Here's how the part is built. I have some questions about the finished solid (model axes, mm). A direction names the side the tool comes from. Coordinates: 2 decimals unless noted, no trailing zeros. Write each loop counter-clockwise with the first axis right and the second up, starting at its lowest first coordinate (ties: lowest second). Pieces come first, ordered by that corner, then holes. Notation, with made-up numbers: M 20,-38.5 L 36,-38.5 A12 cw 36,-18.5 Z; hole C -34.5,-5 d3. An arc over 180 degrees is marked long. Use a Markdown table: item, result.
```python
from build123d import *

# Parameters (mm, degrees)
BOSS_EXTRUDE1_DEPTH       = 46
SKETCH3_W                 = 25
SKETCH3_H                 = 25
BOSS_EXTRUDE2_DEPTH       = 2
SKETCH4_R                 = 1.25
SKETCH4_R_2               = 5
CUT_EXTRUDE1_DEPTH        = 3
FILLET1_R                 = 10
SKETCH5_R                 = 2
CUT_EXTRUDE2_DEPTH        = 26
LPATTERN1_COUNT           = 4
LPATTERN1_PITCH           = 10
LPATTERN1_COPY_1_SKETCH_R = 2
LPATTERN1_COPY_1_DEPTH    = 26
LPATTERN1_COPY_2_SKETCH_R = 2
LPATTERN1_COPY_2_DEPTH    = 26
LPATTERN1_COPY_3_SKETCH_R = 2
LPATTERN1_COPY_3_DEPTH    = 26


with BuildPart() as part:
    # Sketch2 → Boss-Extrude1 (new body)
    with BuildSketch(Plane.XY):
        with BuildLine():
            Line((-12.5, -3.978039328), (12.5, -3.978039328))
            Line((12.5, -3.978039328), (12.468421549, 6.021910812))
            Line((12.468421549, 6.021910812), (10.968421549, 6.021910812))
            ThreePointArc((10.968421549, 6.021910812), (0, 0), (-10.968421549, 6.021910812))
            Line((-10.968421549, 6.021910812), (-12.468421549, 6.021910812))
            Line((-12.468421549, 6.021910812), (-12.5, -3.978039328))
        make_face()
    extrude(amount=BOSS_EXTRUDE1_DEPTH)

    # Sketch3 → Boss-Extrude2 (add)
    with BuildSketch(Plane(origin=(0, 0, 0), x_dir=(-1, 0, 0), z_dir=(0, 0, -1))):
        with Locations((0, 8.521960672)):
            Rectangle(SKETCH3_W, SKETCH3_H)
    extrude(amount=BOSS_EXTRUDE2_DEPTH)

    # Sketch4 → Cut-Extrude1 (cut, through all)
    with BuildSketch(Plane.XY):
        with Locations((-9.5, 13)):
            Circle(SKETCH4_R)
        with Locations((9.5, 13)):
            Circle(SKETCH4_R)
        with Locations((0, 10)):
            Circle(SKETCH4_R_2)
    extrude(amount=-CUT_EXTRUDE1_DEPTH, mode=Mode.SUBTRACT)

    # Fillet1
    fillet1_edges = [part.edges().sort_by_distance(p)[0] for p in [
        (12.5, 21.021960672, -1),
        (-12.5, 21.021960672, -1),
    ]]
    fillet(fillet1_edges, radius=FILLET1_R)

    # Sketch5 → Cut-Extrude2 (cut, through all)
    with BuildSketch(Plane.XZ.offset(3.978039328)):
        with Locations((-8.5, 8)):
            Circle(SKETCH5_R)
    cut_extrude2 = extrude(amount=-CUT_EXTRUDE2_DEPTH, mode=Mode.SUBTRACT)

    # Mirror1: Cut-Extrude2 across plane
    add(cut_extrude2.mirror(Plane(origin=(0, 0, 0), x_dir=(0, 0, 1), z_dir=(1, 0, 0))), mode=Mode.SUBTRACT)

    # LPattern1: Cut-Extrude2 ×4
    with Locations(*[(0, 0, i * LPATTERN1_PITCH) for i in range(1, LPATTERN1_COUNT)]):
        add(cut_extrude2, mode=Mode.SUBTRACT)

    # LPattern1 copy 1 sketch → LPattern1 copy 1 (cut, through all)
    with BuildSketch(Plane(origin=(0, -3.978039328, 10), x_dir=(-1, 0, 0), z_dir=(0, -1, 0))):
        with Locations((-8.5, -8)):
            Circle(LPATTERN1_COPY_1_SKETCH_R)
    extrude(amount=-LPATTERN1_COPY_1_DEPTH, mode=Mode.SUBTRACT)

    # LPattern1 copy 2 sketch → LPattern1 copy 2 (cut, through all)
    with BuildSketch(Plane(origin=(0, -3.978039328, 20), x_dir=(-1, 0, 0), z_dir=(0, -1, 0))):
        with Locations((-8.5, -8)):
            Circle(LPATTERN1_COPY_2_SKETCH_R)
    extrude(amount=-LPATTERN1_COPY_2_DEPTH, mode=Mode.SUBTRACT)

    # LPattern1 copy 3 sketch → LPattern1 copy 3 (cut, through all)
    with BuildSketch(Plane(origin=(0, -3.978039328, 30), x_dir=(-1, 0, 0), z_dir=(0, -1, 0))):
        with Locations((-8.5, -8)):
            Circle(LPATTERN1_COPY_3_SKETCH_R)
    extrude(amount=-LPATTERN1_COPY_3_DEPTH, mode=Mode.SUBTRACT)


solid = part.part
```
1. We'd pull the mould along X, two halves only. Please class faces 4 (the face through (0, 21.022, -1)), 5 (the face through (-10.421, 13.845, -0.986)), 6 (the face through (-9.493, 18.17, -1.014)), 7 (the face through (9.648, 18.015, -1.014)): +X half, -X half, draft (parallel to the pull), parting line (faces both ways), or undercut.
Answers follow:
| item | result |
|---|---|
| face 4 | draft |
| face 5 | undercut |
| face 6 | -X half |
| face 7 | +X half |
2. Suppose I cut it at C-C on z = 38. Write out the boundary of the cut face in (x, y), and give its area (3 significant figures).
Answers follow:
| item | result |
|---|---|
| outline | M -12.5,-3.98 L -10.5,-3.98 L -10.5,5.34 A13 cw -10.97,6.02 L -12.47,6.02 Z; M -6.5,-3.98 L 6.5,-3.98 L 6.5,1.74 A13 cw -6.5,1.74 Z; M 10.5,-3.98 L 12.5,-3.98 L 12.47,6.02 L 10.97,6.02 A13 cw 10.5,5.34 Z |
| area | 98.4 mm2 |
3. Suppose I cut it at D-D on y = -1.5. State how many separate pieces and enclosed holes the cut face has, and give its area (3 significant figures).
Answers follow:
| item | result |
|---|---|
| separate pieces | 1 |
| enclosed holes | 8 |
| area | 1,100 mm2 |
4. Suppose I cut it at B-B on y = 7.75. Write out the boundary of the cut face in (x, z).
Answers follow:
| item | result |
|---|---|
| outline | M -12.5,-2 L -4.47,-2 L -4.47,0 L -12.5,0 Z; M 4.47,-2 L 12.5,-2 L 12.5,0 L 4.47,0 Z |
5. Suppose I cut it at A-A on x = 0. Write out the boundary of the cut face in (y, z).
Answers follow:
| item | result |
|---|---|
| outline | M -3.98,-2 L 5,-2 L 5,0 L 0,0 L 0,46 L -3.98,46 Z; M 15,-2 L 21.02,-2 L 21.02,0 L 15,0 Z |
6. Will these pins go through, and if not, where does the flat tip stop? pin 1 Ø6 at (y, z) = (6.5, 28) entering from -X; pin 2 Ø1.6 at (x, z) = (-11.5, 30.5) entering from +Y; pin 3 Ø13 at (x, y) = (0, 10) entering from +Z.
Answers follow:
| item | result |
|---|---|
| pin 1 | stops at x = -12.48 |
| pin 2 | stops at y = 6.02 |
| pin 3 | stops at z = 0 |
7. I need wall thicknesses on probe 1 along X at (y, z) = (-1.25, 28); probe 2 along Z at (x, y) = (8.5, 2); probe 3 along X at (y, z) = (1.25, 28). Which ranges of each line are inside material? Lowest first, please.
Answers follow:
| item | result |
|---|---|
| probe 1 | x = -12.49 to -10.5, -6.5 to 6.5, 10.5 to 12.49 |
| probe 2 | z = -2 to 6, 10 to 16, 20 to 26, 30 to 36, 40 to 46 |
| probe 3 | x = -12.48 to -10.5, -6.5 to -5.56, 5.56 to 6.5, 10.5 to 12.48 |
8. Which directions (+Z, -Z, +X, -X, +Y, -Y) give clear straight access to the entire face, cutting with the end or side of a thin tool? Please do faces 1 (the face through (3, 14.3, 0)), 2 (the face through (10.498, -0.421, 17.912)), 3 (the face through (12, 6.022, 23)).
Answers follow:
| item | result |
|---|---|
| face 1 | +Z, +Y |
| face 2 | +Y, -Y |
| face 3 | +Z, +X, -X, +Y |
